The listing builds one solid part. Answer for the finished solid, in the listing's coordinates (mm). Face numbers are marked on the shaded views. Round coordinates to 2 decimals unless told otherwise and drop trailing zeros. Write each loop counter-clockwise with the first axis right and the second up, starting at its lowest first coordinate (ties: lowest second). Pieces come first, ordered by that corner, then holes.
(1) The mould has two halves that part along X. Classify the marked faces 1, 2 and 3: +X half, -X half, draft (parallel to the pull), parting line (faces both ways), or undercut.
(2) A cutting plane is placed at B-B, the plane z = 0. Give the vertices of the cut face in (x, y) (3 decimals).
(3) A cutting plane is placed at A-A, the plane x = 0. Give the vertices of the cut face in (y, z) (3 decimals), and give its area (3 significant figures).
(4) Each of these flat-tipped pins is pushed along its axis until it touches: pin 1 Ø1.7 at (x, z) = (-0.5, -19.5) entering from +Y (3 decimals); pin 2 Ø1 at (y, z) = (-4, 13.5) entering from -X; pin 3 Ø1 at (y, z) = (4, 3) entering from -X. Where does it stop, or does it pass through?
(5) A cutting plane is placed at C-C, the plane x = -15. Give the number of separate pieces and of enclosed holes in the cut face, and give its area (3 significant figures).
(6) Find the intervals of material crossed by probe 1 along Y at (x, z) = (-19, -10) (3 decimals); probe 2 along Y at (x, z) = (-12, -7.5); probe 3 along Z at (x, y) = (-16, -4), in increasing order.
from build123d import *

# Parameters (mm, degrees)
BOSS_EXTRUDE1_DEPTH = 3.175
BOSS_EXTRUDE2_DEPTH = 3.175
SKETCH3_R           = 19.05
SKETCH3_R_2         = 15.875
BOSS_EXTRUDE3_DEPTH = 6.35
SKETCH4_R           = 2.54
CUT_EXTRUDE1_DEPTH  = 34.89972345
CHAMFER1_SIZE       = 1.27
SKETCH5_R           = 9.525
CUT_EXTRUDE2_DEPTH  = 34.89972345


with BuildPart() as part:
    # Sketch1 → Boss-Extrude1 (new body)
    with BuildSketch(Plane(origin=(0, 0, 0), x_dir=(1, 0, 0), z_dir=(0, 1, 0))):
        with BuildLine():
            Line((-15.875, -22.225), (15.875, -22.225))
            ThreePointArc((15.875, -22.225), (20.365128061, -20.365128061), (22.225, -15.875))
            Line((22.225, -15.875), (22.225, 15.875))
            ThreePointArc((22.225, 15.875), (20.365128061, 20.365128061), (15.875, 22.225))
            Line((15.875, 22.225), (-15.875, 22.225))
            ThreePointArc((-15.875, 22.225), (-20.365128061, 20.365128061), (-22.225, 15.875))
            Line((-22.225, 15.875), (-22.225, -15.875))
            ThreePointArc((-22.225, -15.875), (-20.365128061, -20.365128061), (-15.875, -22.225))
        make_face()
    extrude(amount=BOSS_EXTRUDE1_DEPTH)

    # Sketch2 → Boss-Extrude2 (add)
    with BuildSketch(Plane(origin=(0, 3.175, 0), x_dir=(1, 0, 0), z_dir=(0, 1, 0))):
        with BuildLine():
            Line((9.779188038, 17.653644576), (-8.104452463, 17.653644576))
            ThreePointArc((-8.104452463, 17.653644576), (-9.392376749, 18.004386475), (-10.324608902, 18.959746126))
            ThreePointArc((-10.324608902, 18.959746126), (-12.655189283, 21.348145252), (-15.875, 22.225))
            ThreePointArc((-15.875, 22.225), (-20.365128061, 20.365128061), (-22.225, 15.875))
            ThreePointArc((-22.225, 15.875), (-21.348011707, 12.654962289), (-18.959285714, 10.324353044))
            ThreePointArc((-18.959285714, 10.324353044), (-18.003795317, 9.392109345), (-17.653, 8.104094261))
            Line((-17.653, 8.104094261), (-17.653, -8.104094261))
            ThreePointArc((-17.653, -8.104094261), (-18.003795317, -9.392109345), (-18.959285714, -10.324353044))
            ThreePointArc((-18.959285714, -10.324353044), (-21.348011707, -12.654962289), (-22.225, -15.875))
            ThreePointArc((-22.225, -15.875), (-20.365128061, -20.365128061), (-15.875, -22.225))
            ThreePointArc((-15.875, -22.225), (-12.655189283, -21.348145252), (-10.324608902, -18.959746126))
            ThreePointArc((-10.324608902, -18.959746126), (-9.392376749, -18.004386475), (-8.104452463, -17.653644576))
            Line((-8.104452463, -17.653644576), (8.104452463, -17.653644576))
            ThreePointArc((8.104452463, -17.653644576), (9.392376749, -18.004386475), (10.324608902, -18.959746126))
            ThreePointArc((10.324608902, -18.959746126), (12.655189283, -21.348145252), (15.875, -22.225))
            ThreePointArc((15.875, -22.225), (20.365128061, -20.365128061), (22.225, -15.875))
            ThreePointArc((22.225, -15.875), (21.348011707, -12.654962289), (18.959285714, -10.324353044))
            ThreePointArc((18.959285714, -10.324353044), (18.003795317, -9.392109345), (17.653, -8.104094261))
            Line((17.653, -8.104094261), (17.653, 8.104094261))
            ThreePointArc((17.653, 8.104094261), (18.003795317, 9.392109345), (18.959285714, 10.324353044))
            ThreePointArc((18.959285714, 10.324353044), (21.348011707, 12.654962289), (22.225, 15.875))
            ThreePointArc((22.225, 15.875), (20.365128061, 20.365128061), (15.875, 22.225))
            ThreePointArc((15.875, 22.225), (12.065268583, 20.955201426), (9.779188038, 17.653644576))
        make_face()
    extrude(amount=BOSS_EXTRUDE2_DEPTH)

    # Sketch3 → Boss-Extrude3 (add)
    with BuildSketch(Plane.XZ):
        with Locations(Location((0, 0, 0), (0, 0, 90))):
            Circle(SKETCH3_R)
        with Locations(Location((0, 0, 0), (0, 0, 270))):
            Circle(SKETCH3_R_2, mode=Mode.SUBTRACT)
    extrude(amount=BOSS_EXTRUDE3_DEPTH)

    # Sketch4 → Cut-Extrude1 (cut, through all)
    with BuildSketch(Plane(origin=(0, 6.35, 0), x_dir=(1, 0, 0), z_dir=(0, 1, 0))):
        with Locations(Location((-15.875, 15.639418556, 0), (0, 0, 270))):
            Circle(SKETCH4_R)
        with Locations(Location((15.875, 15.639418556, 0), (0, 0, 270))):
            Circle(SKETCH4_R)
        with Locations(Location((-15.875, -15.639418556, 0), (0, 0, 270))):
            Circle(SKETCH4_R)
        with Locations(Location((15.875, -15.639418556, 0), (0, 0, 270))):
            Circle(SKETCH4_R)
    extrude(amount=-CUT_EXTRUDE1_DEPTH, mode=Mode.SUBTRACT)

    # Chamfer1
    chamfer1_edges = [part.edges().sort_by_distance(p)[0] for p in [
        (-20.365314283, 6.35, -20.36494183),
        (-20.365314283, 6.35, 20.36494183),
        (-9.392376749, 6.35, -18.004386475),
        (19.836937806, 6.35, -20.837413609),
        (0.837367788, 6.35, -17.653644576),
        (18.003795317, 6.35, -9.392109345),
        (17.653, 6.35, 0),
        (18.003795317, 6.35, 9.392109345),
        (-18.003795317, 6.35, -9.392109345),
        (20.365314283, 6.35, 20.36494183),
        (-17.653, 6.35, 0),
        (9.392376749, 6.35, 18.004386475),
        (-18.003795317, 6.35, 9.392109345),
        (0, 6.35, 17.653644576),
        (-9.392376749, 6.35, 18.004386475),
    ]]
    chamfer(chamfer1_edges, length=CHAMFER1_SIZE)
    chamfer1_2_edges = [part.edges().sort_by_distance(p)[0] for p in [
        (0, -6.35, -19.05),
    ]]
    chamfer(chamfer1_2_edges, length=CHAMFER1_SIZE)
    chamfer1_3_edges = [part.edges().sort_by_distance(p)[0] for p in [
        (0, -6.35, 15.875),
    ]]
    chamfer(chamfer1_3_edges, length=CHAMFER1_SIZE)
    # the kernel refuses this chamfer: 1.27 mm, written as the material it takes off along each edge
    with BuildSketch(Plane(origin=(-22.225, 3.175, -19.141037395), x_dir=(-0.02749587661058728, -0.9996219169112966, 0), z_dir=(0, 0, 1))) as chamfer1_4_piece_1_section:
        with BuildLine():
            Line((1.306414958, 0), (-0.071814887, 1.304439598))
            Line((-0.071814887, 1.304439598), (-0.097205283, 1.303741203))
            ThreePointArc((-0.097205283, 1.303741203), (-0.043344118, 0.652015244), (-0.025390397, -0.000698395))
            Line((-0.025390397, -0.000698395), (0.000698395, -0.025390397))
            ThreePointArc((0.000698395, -0.025390397), (0.653412034, -0.007436675), (1.307113353, -0.025390397))
            Line((1.307113353, -0.025390397), (1.306414958, 0))
        make_face()
    chamfer1_4_piece_1 = extrude(amount=38.282074789, mode=Mode.PRIVATE)
    chamfer1_4_piece_1 = chamfer1_4_piece_1 - Plane(origin=(-15.875, 2.735416382, -15.875), x_dir=(0, 0, -1), z_dir=(0, -1, 0)) * Cylinder(6.35, 82, mode=Mode.PRIVATE)
    chamfer1_4_piece_1 = chamfer1_4_piece_1 - Plane(origin=(-15.875, 2.735416382, 15.875), x_dir=(-1, 0, 0), z_dir=(0, -1, 0)) * Cylinder(6.35, 82, mode=Mode.PRIVATE)
    add(chamfer1_4_piece_1, mode=Mode.SUBTRACT)
    # the kernel refuses this chamfer: 1.27 mm, written as the material it takes off along each edge
    with BuildSketch(Plane(origin=(19.141037395, 3.175, -22.225), x_dir=(0, -0.9996219169112966, -0.02749587661058728), z_dir=(-1, 0, 0))) as chamfer1_5_piece_1_section:
        with BuildLine():
            Line((1.306414958, 0), (-0.071814887, 1.304439598))
            Line((-0.071814887, 1.304439598), (-0.097205283, 1.303741203))
            ThreePointArc((-0.097205283, 1.303741203), (-0.043344118, 0.652015244), (-0.025390397, -0.000698395))
            Line((-0.025390397, -0.000698395), (0.000698395, -0.025390397))
            ThreePointArc((0.000698395, -0.025390397), (0.653412034, -0.007436675), (1.307113353, -0.025390397))
            Line((1.307113353, -0.025390397), (1.306414958, 0))
        make_face()
    chamfer1_5_piece_1 = extrude(amount=38.282074789, mode=Mode.PRIVATE)
    chamfer1_5_piece_1 = chamfer1_5_piece_1 - Plane(origin=(-15.875, 2.735416382, -15.875), x_dir=(0, 0, -1), z_dir=(0, -1, 0)) * Cylinder(6.35, 82, mode=Mode.PRIVATE)
    chamfer1_5_piece_1 = chamfer1_5_piece_1 - Plane(origin=(15.875, 2.735416382, -15.875), x_dir=(1, 0, 0), z_dir=(0, -1, 0)) * Cylinder(6.35, 82, mode=Mode.PRIVATE)
    add(chamfer1_5_piece_1, mode=Mode.SUBTRACT)
    # the kernel refuses this chamfer: 1.27 mm, written as the material it takes off along each edge
    with BuildSketch(Plane(origin=(-19.141037395, 3.175, 22.225), x_dir=(0, -0.9996219169112966, 0.02749587661058728), z_dir=(1, 0, 0))) as chamfer1_6_piece_1_section:
        with BuildLine():
            Line((1.306414958, 0), (-0.071814887, 1.304439598))
            Line((-0.071814887, 1.304439598), (-0.097205283, 1.303741203))
            ThreePointArc((-0.097205283, 1.303741203), (-0.043344118, 0.652015244), (-0.025390397, -0.000698395))
            Line((-0.025390397, -0.000698395), (0.000698395, -0.025390397))
            ThreePointArc((0.000698395, -0.025390397), (0.653412034, -0.007436675), (1.307113353, -0.025390397))
            Line((1.307113353, -0.025390397), (1.306414958, 0))
        make_face()
    chamfer1_6_piece_1 = extrude(amount=38.282074789, mode=Mode.PRIVATE)
    chamfer1_6_piece_1 = chamfer1_6_piece_1 - Plane(origin=(-15.875, 2.735416383, 15.875), x_dir=(-1, 0, 0), z_dir=(0, -1, 0)) * Cylinder(6.35, 82, mode=Mode.PRIVATE)
    chamfer1_6_piece_1 = chamfer1_6_piece_1 - Plane(origin=(15.875, 2.735416383, 15.875), x_dir=(0, 0, 1), z_dir=(0, -1, 0)) * Cylinder(6.35, 82, mode=Mode.PRIVATE)
    add(chamfer1_6_piece_1, mode=Mode.SUBTRACT)
    # the kernel refuses this chamfer: 1.27 mm, written as the material it takes off along each edge
    with BuildSketch(Plane(origin=(22.225, 3.175, 19.141037395), x_dir=(0.02749587661058728, -0.9996219169112966, 0), z_dir=(0, 0, -1))) as chamfer1_7_piece_1_section:
        with BuildLine():
            Line((1.306414958, 0), (-0.071814887, 1.304439598))
            Line((-0.071814887, 1.304439598), (-0.097205283, 1.303741203))
            ThreePointArc((-0.097205283, 1.303741203), (-0.043344118, 0.652015244), (-0.025390397, -0.000698395))
            Line((-0.025390397, -0.000698395), (0.000698395, -0.025390397))
            ThreePointArc((0.000698395, -0.025390397), (0.653412034, -0.007436675), (1.307113353, -0.025390397))
            Line((1.307113353, -0.025390397), (1.306414958, 0))
        make_face()
    chamfer1_7_piece_1 = extrude(amount=38.282074789, mode=Mode.PRIVATE)
    chamfer1_7_piece_1 = chamfer1_7_piece_1 - Plane(origin=(15.875, 2.735416383, -15.875), x_dir=(1, 0, 0), z_dir=(0, -1, 0)) * Cylinder(6.35, 82, mode=Mode.PRIVATE)
    chamfer1_7_piece_1 = chamfer1_7_piece_1 - Plane(origin=(15.875, 2.735416383, 15.875), x_dir=(0, 0, 1), z_dir=(0, -1, 0)) * Cylinder(6.35, 82, mode=Mode.PRIVATE)
    add(chamfer1_7_piece_1, mode=Mode.SUBTRACT)

    # Sketch5 → Cut-Extrude2 (cut, through all)
    with BuildSketch(Plane(origin=(0, 6.35, 0), x_dir=(1, 0, 0), z_dir=(0, 1, 0))):
        with Locations(Location((0, 0, 0), (0, 0, 270))):
            Circle(SKETCH5_R)
    extrude(amount=-CUT_EXTRUDE2_DEPTH, mode=Mode.SUBTRACT)


solid = part.part
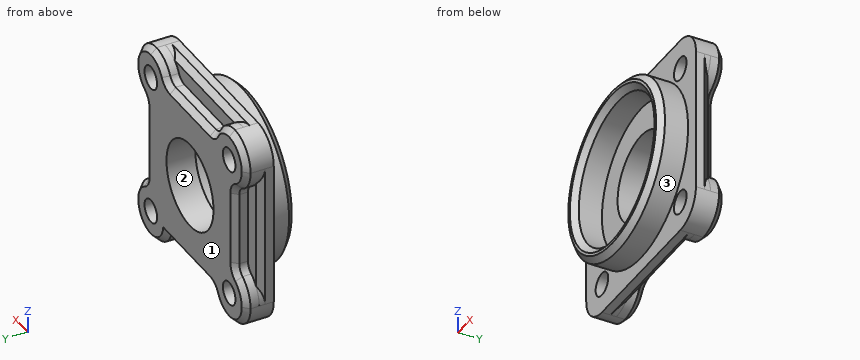
Solutions:
1. face 1: draft
1. face 2: undercut
1. face 3: parting line
2. outline: (-22.225, 0) - (-19.05, 0) - (-19.05, -5.08) - (-17.78, -6.35) - (-17.145, -6.35) - (-15.875, -5.08) - (-15.875, 0) - (-9.525, 0) - (-9.525, 6.35) - (-16.383, 6.35) - (-17.653, 5.08) - (-17.653, 3.175) - (-20.955, 3.175) - (-22.225, 1.905) - close; (9.525, 0) - (15.875, 0) - (15.875, -5.08) - (17.145, -6.35) - (17.78, -6.35) - (19.05, -5.08) - (19.05, 0) - (22.225, 0) - (22.225, 1.905) - (20.955, 3.175) - (17.653, 3.175) - (17.653, 5.08) - (16.383, 6.35) - (9.525, 6.35) - close
3. outline: (-6.35, -17.78) - (-5.08, -19.05) - (0, -19.05) - (0, -22.225) - (1.905, -22.225) - (3.175, -20.955) - (3.175, -17.654) - (5.08, -17.654) - (6.35, -16.384) - (6.35, -9.525) - (0, -9.525) - (0, -15.875) - (-5.08, -15.875) - (-6.35, -17.145) - close; (-6.35, 17.145) - (-5.08, 15.875) - (0, 15.875) - (0, 9.525) - (6.35, 9.525) - (6.35, 16.384) - (5.08, 17.654) - (3.175, 17.654) - (3.175, 20.955) - (1.905, 22.225) - (0, 22.225) - (0, 19.05) - (-5.08, 19.05) - (-6.35, 17.78) - close
3. area: 166 mm2
4. pin 1: stops at y = 3.175
4. pin 2: stops at x = -13.92
4. pin 3: stops at x = -17.65
5. separate pieces: 3
5. enclosed holes: 0
5. area: 296 mm2
6. probe 1: y = 0 to 3.175
6. probe 2: y = 0 to 6.35
6. probe 3: z = -10.34 to 10.34
